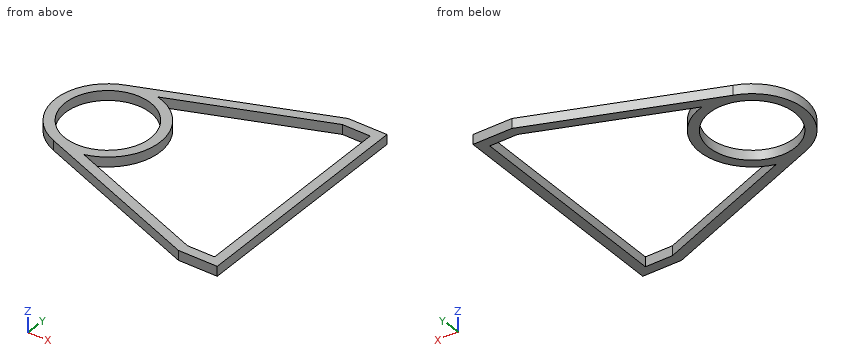
```python
from build123d import *

# Parameters (mm, degrees)
F0_W     = 6.35
F0_H     = 6.35
F0_H_2   = 69.85
F1_DEPTH = 6.35
F2_R     = 27.94
F3_DEPTH = 25.4
F5_DEPTH = 25.4


with BuildPart() as f1:
    # F0 (on Top) → F1 (new body)
    with BuildSketch(Plane.XY):
        with Locations((66.649964, 62.1324)):
            Rectangle(F0_W, F0_H)
        with Locations((66.649964, 24.0324)):
            Rectangle(F0_W, F0_H_2)
        with BuildLine():
            Line((63.474964, 58.9574), (63.474964, 65.3074))
            Line((63.474964, 65.3074), (44.424964, 65.3074))
            Line((44.424964, 65.3074), (-68.375352, 21.516612))
            ThreePointArc((-68.375352, 21.516612), (-91.459051, -10.251982), (-69.578284, -42.860765))
            Line((-69.578284, -42.860765), (44.424964, -87.0926))
            Line((44.424964, -87.0926), (63.474964, -87.0926))
            Line((63.474964, -87.0926), (63.474964, -80.7426))
            Line((63.474964, -80.7426), (63.474964, -10.8926))
            Line((63.474964, -10.8926), (63.474964, 58.9574))
        make_face()
        with Locations((66.649964, -45.8176)):
            Rectangle(F0_W, F0_H_2)
        with Locations((66.649964, -83.9176)):
            Rectangle(F0_W, F0_H)
    extrude(amount=F1_DEPTH)

    # F2 (on face) → F3 (cut)
    with BuildSketch(Plane.XY.offset(6.35)):
        with Locations((-57.175036, -10.8926)):
            Circle(F2_R)
    extrude(amount=-F3_DEPTH, mode=Mode.SUBTRACT)

    # F4 (on Top) → F5 (cut)
    with BuildSketch(Plane.XY):
        with BuildLine():
            Line((63.474964, -80.7426), (63.474964, 58.9574))
            Line((63.474964, 58.9574), (45.235226, 58.9574))
            Line((45.235226, 58.9574), (-48.786443, 22.355491))
            ThreePointArc((-48.786443, 22.355491), (-22.885047, -10.86449), (-48.731942, -44.126894))
            Line((-48.731942, -44.126894), (45.783264, -80.7426))
            Line((45.783264, -80.7426), (63.474964, -80.7426))
        make_face()
    extrude(amount=F5_DEPTH, mode=Mode.SUBTRACT)


solid = f1.part
```
Verification items for the finished model (mm, model axes). Round coordinates to 2 decimals unless told otherwise and drop trailing zeros. Loops run counter-clockwise (first coordinate to the right, second up) from the corner with the lowest first, then second, coordinate; pieces in that order, holes last. Notation, with made-up numbers: (-4.5, 58) -> (41.5, 58) arc R10 cw to (41.5, 74) -> close; hole circle Ø11 at (-5.75, 78). An arc over 180 degrees is marked (long way). Answer as a JSON object with one key per item and string values.
Q1. Section check C-C (x = -1). Record the boundary of the cut face in (y, z).
Data:
{"outline": "(-69.47, 0) -> (-62.62, 0) -> (-62.62, 6.35) -> (-69.47, 6.35) -> close; (40.96, 0) -> (47.67, 0) -> (47.67, 6.35) -> (40.96, 6.35) -> close"}
Q2. Go/stop test with flat-tipped pins: P1, Ø6, axis at x = 3.5, y = -59.5, coming from the -Z side; P2, Ø1.9, axis at y = -20, z = 1.5, coming from the -X side; P3, Ø3, axis at x = 42, z = 2.5, coming from the +Y side; P4, Ø3, axis at x = -59, z = 5.5, coming from the +Y side. Record where each tip stops, or that it passes through.
Data:
{"P1": "passes through", "P2": "stops at x = -90.48", "P3": "stops at y = 64.95", "P4": "stops at y = 25.74"}
Q3. Section check B-B (x = -40). Record the boundary of the cut face in (y, z).
Data:
{"outline": "(-54.34, 0) -> (-47.51, 0) -> (-47.51, 6.35) -> (-54.34, 6.35) -> close; (-40.57, 0) -> (-32.93, 0) -> (-32.93, 6.35) -> (-40.57, 6.35) -> close; (11.15, 0) -> (18.79, 0) -> (18.79, 6.35) -> (11.15, 6.35) -> close; (25.78, 0) -> (32.53, 0) -> (32.53, 6.35) -> (25.78, 6.35) -> close"}
Q4. Scan lines: line 1 (Y direction, x = 58, z = 5); line 2 (X direction, y = -15.5, z = 5); line 3 (X direction, y = -6, z = 1.5). Record each from-to range of solid material in increasing order. Write a range as from..to.
Data:
{"line 1": "y = -87.09..-80.74, 58.96..65.31", "line 2": "x = -91.15..-84.73, -29.62..-23.2, 63.47..69.82", "line 3": "x = -91.11..-84.68, -29.67..-23.24, 63.47..69.82"}
Q5. Section check D-D (y = -35). Record the boundary of the cut face in (x, z), then the cut area to 3 significant figures.
Data:
{"outline": "(-81.56, 0) -> (-71.3, 0) -> (-71.3, 6.35) -> (-81.56, 6.35) -> close; (-43.05, 0) -> (-32.79, 0) -> (-32.79, 6.35) -> (-43.05, 6.35) -> close; (63.47, 0) -> (69.82, 0) -> (69.82, 6.35) -> (63.47, 6.35) -> close", "area": "171 mm2"}
Q6. Section check A-A (y = 40). Record the boundary of the cut face in (x, z), then the cut area to 3 significant figures.
Data:
{"outline": "(-20.76, 0) -> (-3.46, 0) -> (-3.46, 6.35) -> (-20.76, 6.35) -> close; (63.47, 0) -> (69.82, 0) -> (69.82, 6.35) -> (63.47, 6.35) -> close", "area": "150 mm2"}
